from build123d import *

# Parameters (mm, degrees)
CROQUIS1_R                                           = 55
CROQUIS1_R_2                                         = 52.5
SALIENTE_EXTRUIR1_DEPTH                              = 22.5
CROQUIS2_R                                           = 55
SALIENTE_EXTRUIR2_DEPTH                              = 5
REFRENTADO_PARA_TORNILLO_TAP_N_CON_CABEZ_D           = 5.5
REFRENTADO_PARA_TORNILLO_TAP_N_CON_CABEZ_CSINK_D     = 11.2
REFRENTADO_PARA_TORNILLO_TAP_N_CON_CABEZ_CSINK_ANGLE = 90
SALIENTE_EXTRUIR8_DEPTH                              = 10
CROQUIS12_R                                          = 3
CROQUIS12_R_2                                        = 4
CORTAR_EXTRUIR4_DEPTH                                = 10
CORTAR_EXTRUIR6_DEPTH                                = 3
CROQUIS16_R                                          = 1.75
CORTAR_EXTRUIR7_DEPTH                                = 5


with BuildPart() as part:
    # Croquis1 → Saliente-Extruir1 (new body)
    with BuildSketch(Plane.XY):
        Circle(CROQUIS1_R)
        Circle(CROQUIS1_R_2, mode=Mode.SUBTRACT)
    extrude(amount=SALIENTE_EXTRUIR1_DEPTH)

    # Croquis2 → Saliente-Extruir2 (add)
    with BuildSketch(Plane.XY.offset(22.5)):
        Circle(CROQUIS2_R)
    extrude(amount=SALIENTE_EXTRUIR2_DEPTH)

    # Refrentado para tornillo tapón con cabeza plana de clavija de M51 (through all)
    with Locations(Plane.XY.offset(27.5)):
        with Locations((0, 13.5), (-11.691342951, -6.75), (11.691342951, -6.75)):
            CounterSinkHole(REFRENTADO_PARA_TORNILLO_TAP_N_CON_CABEZ_D / 2, REFRENTADO_PARA_TORNILLO_TAP_N_CON_CABEZ_CSINK_D / 2, counter_sink_angle=REFRENTADO_PARA_TORNILLO_TAP_N_CON_CABEZ_CSINK_ANGLE)

    # Croquis10 → Saliente-Extruir8 (add)
    with BuildSketch(Plane(origin=(0, 0, 22.5), x_dir=(-1, 0, 0), z_dir=(0, 0, -1))):
        with BuildLine():
            Line((-3.5, 45), (-3.5, 51))
            ThreePointArc((-3.5, 51), (0, 54.5), (3.5, 51))
            Line((3.5, 51), (3.5, 45))
            ThreePointArc((3.5, 45), (0, 41.5), (-3.5, 45))
        make_face()
        with BuildLine():
            Line((40.72114317, -19.468911087), (45.917295593, -22.468911087))
            ThreePointArc((45.917295593, -22.468911087), (47.198384506, -27.25), (42.417295593, -28.531088913))
            Line((42.417295593, -28.531088913), (37.22114317, -25.531088913))
            ThreePointArc((37.22114317, -25.531088913), (35.940054257, -20.75), (40.72114317, -19.468911087))
        make_face()
        with BuildLine():
            Line((-37.22114317, -25.531088913), (-42.417295593, -28.531088913))
            ThreePointArc((-42.417295593, -28.531088913), (-47.198384506, -27.25), (-45.917295593, -22.468911087))
            Line((-45.917295593, -22.468911087), (-40.72114317, -19.468911087))
            ThreePointArc((-40.72114317, -19.468911087), (-35.940054257, -20.75), (-37.22114317, -25.531088913))
        make_face()
        with BuildLine():
            Line((-4.5, -50.030679936), (-4.5, -38.370856831))
            ThreePointArc((-4.5, -38.370856831), (0, -33.870856831), (4.5, -38.370856831))
            Line((4.5, -38.370856831), (4.5, -50.030679936))
            ThreePointArc((4.5, -50.030679936), (0, -54.530679936), (-4.5, -50.030679936))
        make_face()
    extrude(amount=SALIENTE_EXTRUIR8_DEPTH)

    # Croquis12 → Cortar-Extruir4 (cut)
    with BuildSketch(Plane.XY.offset(27.5)):
        with Locations((0, 47.5)):
            Circle(CROQUIS12_R)
        with Locations((41.13620668, -23.75)):
            Circle(CROQUIS12_R)
        with Locations((-41.13620668, -23.75)):
            Circle(CROQUIS12_R)
        with Locations((0, -47.5)):
            Circle(CROQUIS12_R_2)
    extrude(amount=-CORTAR_EXTRUIR4_DEPTH, mode=Mode.SUBTRACT)

    # Croquis15 → Cortar-Extruir6 (cut)
    with BuildSketch(Plane.XY.offset(27.5)):
        Polygon((-11.904987742, 45.779484215), (-14.067452684, 48.10479682), (-17.162464942, 47.394703548), (-18.095012258, 44.359297671), (-15.932547316, 42.033985067), (-12.837535058, 42.744078339), align=None)
        Polygon((18.095012258, 44.359297671), (15.932547316, 42.033985067), (12.837535058, 42.744078339), (11.904987742, 45.779484215), (14.067452684, 48.10479682), (17.162464942, 47.394703548), align=None)
        Polygon((44.368772548, -7.21900181), (43.436225232, -10.254407687), (45.598690174, -12.579720292), (48.693702432, -11.869627019), (49.626249748, -8.834221143), (47.463784806, -6.508908538), align=None)
        Polygon((34.626249748, -36.235169801), (32.463784806, -38.560482405), (29.368772548, -37.850389133), (28.436225232, -34.814983256), (30.598690174, -32.489670652), (33.693702432, -33.199763924), align=None)
        Polygon((-28.436225232, -34.814983256), (-30.598690174, -32.489670652), (-33.693702432, -33.199763924), (-34.626249748, -36.235169801), (-32.463784806, -38.560482405), (-29.368772548, -37.850389133), align=None)
        Polygon((-48.693702432, -11.869627019), (-49.626249748, -8.834221143), (-47.463784806, -6.508908538), (-44.368772548, -7.21900181), (-43.436225232, -10.254407687), (-45.598690174, -12.579720292), align=None)
    extrude(amount=-CORTAR_EXTRUIR6_DEPTH, mode=Mode.SUBTRACT)

    # Croquis16 → Cortar-Extruir7 (cut)
    with BuildSketch(Plane.XY.offset(27.5)):
        with Locations((-15.003552118, 45.088897544)):
            Circle(CROQUIS16_R)
        with Locations((15.003552118, 45.088897544)):
            Circle(CROQUIS16_R)
        with Locations((46.549906761, -9.55099149)):
            Circle(CROQUIS16_R)
        with Locations((31.546354642, -35.537906053)):
            Circle(CROQUIS16_R)
        with Locations((-31.546354642, -35.537906053)):
            Circle(CROQUIS16_R)
        with Locations((-46.549906761, -9.55099149)):
            Circle(CROQUIS16_R)
    extrude(amount=-CORTAR_EXTRUIR7_DEPTH, mode=Mode.SUBTRACT)


solid = part.part
The listing builds one solid part. Answer for the finished solid, in the listing's coordinates (mm). A direction names the side the tool comes from. Give positions to 0.01 mm unless a question says otherwise; leave off trailing zeros. Loops run counter-clockwise (first coordinate to the right, second up) from the corner with the lowest first, then second, coordinate; pieces in that order, holes last. Notation, with made-up numbers: (63, -31.75) - (97, -31.75) arc R20 ccw to (97, -13.75) - close; hole circle Ø3 at (57.5, 22). An arc over 180 degrees is marked (long way). Write each question's results on one line, items separated by ' | '.
1. Flat-ended cylindrical pins translate along their axes: P1, Ø6, axis at y = -21.5, z = 5.5, coming from the +X side; P2, Ø5, axis at x = -11.69, y = -6.75, coming from the -Z side; P3, Ø2, axis at x = -13, z = 9, coming from the +Y side; P4, Ø4, axis at y = -6.5, z = 8.5, coming from the -X side. Find the tip coordinate at first contact, or state that the pin passes through.
Resolved:
P1: stops at x = 51.8 | P2: passes through | P3: stops at y = 53.67 | P4: stops at x = -54.82
2. Find section A-A, the plane z = 21. Count the separate pieces of the cut face and the enclosed holes in it, then the cut area to 3 significant figures.
Resolved:
separate pieces: 1 | enclosed holes: 5 | area: 1,080 mm^2
3. Find section B-B, the plane x = -21. Write down the section's boundary in (y, z).
Resolved:
outline: (-50.83, 0) - (-48.12, 0) - (-48.12, 22.5) - (48.12, 22.5) - (48.12, 0) - (50.83, 0) - (50.83, 27.5) - (-50.83, 27.5) - close
4. For a pull along Y with two mould halves and no side action, classify faces 4 (the face through (20, -49, 0)), 5 (the face through (45.26, -8.37, 23.51)) as +Y half, -Y half, draft (parallel to the pull), parting line (faces both ways), or undercut.
Resolved:
face 4: draft | face 5: undercut
5. Which of the six approach directions +Z, -Z, +X, -X, +Y, -Y give full straight-line access (tool end or side, diameter ignored) to faces 1 (the face through (30, -37, 24.5)), 2 (the face through (0.358, 16.227, 23.56)), 3 (the face through (43.356, -20.99, 17.57))?
Resolved:
face 1: +Z | face 2: +Z, -Z | face 3: -Z
6. Consider probe 1 along Z at (x, y) = (-25, 16.5); probe 2 along X at (y, z) = (-42, 20.25); probe 3 along X at (y, z) = (13.5, 23.9). Determine where each line is inside the solid, lowest interval first. Write a range as from..to.
Resolved:
probe 1: z = 22.5..27.5 | probe 2: x = -35.51..-31.5, -4.5..4.5, 31.5..35.51 | probe 3: x = -53.32..-2.75, 2.75..53.32
